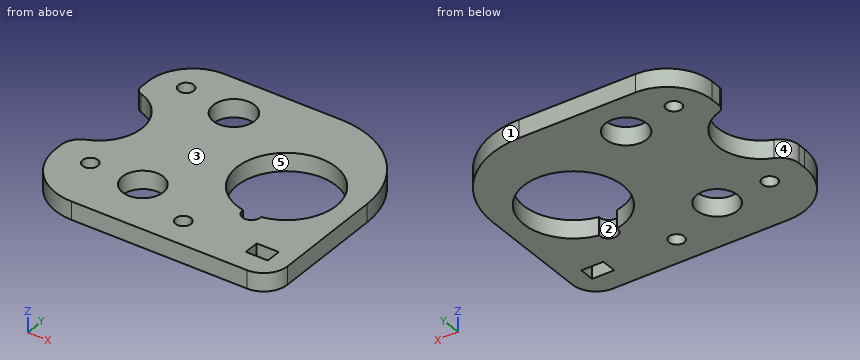
Solid Edge part; units mm, degrees
sketch "Sketch1" plane through (0, 0, 0) normal (0, 0, 1) x (1, 0, 0)
  arc A0 (-24.2481, 16.1032) -> (-14.29, 26.0612) centre (-14.29, 16.1032) cw
  line L0 (-14.29, 26.0612) -> (11.5125, 26.0612)
  arc A1 (11.5125, 26.0612) -> (31.2468, 6.3269) centre (11.5125, 6.3269) cw
  line L1 (31.2468, 6.3269) -> (31.2468, -18.6416)
  arc A2 (31.2468, -18.6416) -> (25.9694, -23.9191) centre (25.9694, -18.6416) cw
  line L2 (25.9694, -23.9191) -> (-12.9101, -23.9191)
  arc A3 (-12.9101, -23.9191) -> (-25.1463, -11.683) centre (-12.9101, -11.683) cw
  line L3 (-25.1463, -11.683) -> (-25.1463, -9.9593)
  arc A4 (-25.1463, -9.9593) -> (-22.3744, -5.9106) centre (-20.8035, -9.9593) cw
  arc A5 (-22.3744, -5.9106) -> (-22.9813, 12.095) centre (-25.8263, 2.9861) ccw
  arc A6 (-22.9813, 12.095) -> (-24.2481, 13.8177) centre (-22.4432, 13.8177) cw
  line L4 (-24.2481, 13.8177) -> (-24.2481, 16.1032)
  circle A7 centre (7.308, -17.457) radius 1.7
  arc A8 (18.0497, -8.2752) -> (14.0663, -8.2752) centre (16.058, -8.457) cw
  arc A9 (14.0663, -8.2752) -> (18.0497, -8.2752) centre (16.058, 2.543) cw
  circle A10 centre (-17.3918, -11.684) radius 1.7
  circle A11 centre (-17.3918, 18.3557) radius 1.7
  line L5 (27.2537, -19.157) -> (22.3605, -19.157)
  line L6 (27.2537, -15.757) -> (27.2537, -19.157)
  line L7 (22.3605, -15.757) -> (27.2537, -15.757)
  line L8 (22.3605, -19.157) -> (22.3605, -15.757)
extrude "Protrusion1" add sketch "Sketch1" against normal blind 4
sketch "Sketch2" plane through (3.0503, 1.0711, -4) normal (0, 0, -1) x (-1, 0, 0)
  circle A0 centre (8.6319, 15.5619) radius 4.5794
  circle A1 centre (8.6229, -13.0011) radius 4.5063
extrude "Cutout1" cut sketch "Sketch2" against normal up to next
Here's how the part is built. I have some questions about the finished solid (model axes, mm). Face numbers are marked on the shaded views. A direction names the side the tool comes from. Round coordinates to 2 decimals unless told otherwise and drop trailing zeros. Loops run counter-clockwise (first coordinate to the right, second up) from the corner with the lowest first, then second, coordinate; pieces in that order, holes last.
1. If we section it at C-C on x = 19: Write out the boundary of the cut face in (y, z), plus the area to 3 significant figures.
Answer list:
outline: (-23.92, -4) - (-8.06, -4) - (-8.06, 0) - (-23.92, 0) - close; (13.14, -4) - (24.59, -4) - (24.59, 0) - (13.14, 0) - close
area: 109 mm2
2. For P1, Ø2, axis at y = 13, z = -3, coming from the +X side; P2, Ø1.8, axis at y = 15.5, z = -2, coming from the -X side; P3, Ø2, axis at y = 2.5, z = -3.5, coming from the -X side, each with a flat end and sliding along its axis, tell me the tip position at first contact or that it passes through.
Answer list:
P1: stops at x = 30.41
P2: stops at x = -24.25
P3: stops at x = -16.4
3. If I drill on line 1 along Y through (x, z) = (-16, -1.1); line 2 along X through (y, z) = (-12, -3.5); line 3 along Y through (x, z) = (-18.5, -1.8), over which ranges is the centre line in solid material (lowest first)?
Answer list:
line 1: y = -23.52 to -12.66, -10.71 to 17.38, 19.33 to 25.91
line 2: x = -25.14 to -19.06, -15.72 to -10.08, -1.07 to 31.25
line 3: y = -22.57 to -12.97, -10.39 to -3.13, 9.1 to 17.07, 19.64 to 25.13
4. If we section it at A-A on x = -18: Write out the boundary of the cut face in (y, z).
Answer list:
outline: (-22.81, -4) - (-13.27, -4) - (-13.27, 0) - (-22.81, 0) - close; (-10.1, -4) - (-2.47, -4) - (-2.47, 0) - (-10.1, 0) - close; (8.45, -4) - (16.77, -4) - (16.77, 0) - (8.45, 0) - close; (19.94, -4) - (25.34, -4) - (25.34, 0) - (19.94, 0) - close
5. If we section it at B-B on y = -9: Write out the boundary of the cut face in (x, z), plus the area to 3 significant figures.
Answer list:
outline: (-25.04, -4) - (-9, -4) - (-9, 0) - (-25.04, 0) - close; (-2.15, -4) - (14.13, -4) - (14.13, 0) - (-2.15, 0) - close; (17.98, -4) - (31.25, -4) - (31.25, 0) - (17.98, 0) - close
area: 182 mm2
6. We'd pull the mould along Y, two halves only. Please class the marked faces 1, 2 and 3: +Y half, -Y half, draft (parallel to the pull), parting line (faces both ways), or undercut.
Answer list:
face 1: +Y half
face 2: undercut
face 3: draft
7. Which directions (+Z, -Z, +X, -X, +Y, -Y) give clear straight access to the entire face, cutting with the end or side of a thin tool? Please do the marked faces 4 and 5.
Answer list:
face 4: +Z, -Z, -X
face 5: +Z, -Z
8. If we section it at D-D on z = -1.95: Write out the boundary of the cut face in (x, y).
Answer list:
outline: (-25.15, -11.68) arc R12.24 ccw to (-12.91, -23.92) - (25.97, -23.92) arc R5.28 ccw to (31.25, -18.64) - (31.25, 6.33) arc R19.73 ccw to (11.51, 26.06) - (-14.29, 26.06) arc R9.96 ccw to (-24.25, 16.1) - (-24.25, 13.82) arc R1.8 ccw to (-22.98, 12.09) arc R9.54 cw to (-22.37, -5.91) arc R4.34 ccw to (-25.15, -9.96) - close; hole circle Ø3.4 at (-17.39, -11.68); hole circle Ø3.4 at (-17.39, 18.36); hole circle Ø9.16 at (-5.58, 16.63); hole circle Ø9.01 at (-5.57, -11.93); hole circle Ø3.4 at (7.31, -17.46); hole (14.07, -8.28) arc R2 ccw (long way) to (18.05, -8.28) arc R11 ccw (long way) to start; hole (22.36, -19.16) - (27.25, -19.16) - (27.25, -15.76) - (22.36, -15.76) - close
